Here's how the part is built. I have some questions about the finished solid (model axes, mm). A direction names the side the tool comes from. Give positions to 0.01 mm unless a question says otherwise; leave off trailing zeros. Write each loop counter-clockwise with the first axis right and the second up, starting at its lowest first coordinate (ties: lowest second). Pieces come first, ordered by that corner, then holes. Notation, with made-up numbers: (-26, 55) -> (-6, 55) arc R31 ccw to (-6, 80) -> close; hole circle Ø1 at (-26, -10.75). An arc over 180 degrees is marked (long way). Put each result on its own line as item: value. Start each with the question number.
Autodesk Inventor part; units mm, degrees
ref_plane "YZ Plane" through (0, 0, 0) normal (1, 0, 0) x (0, 1, 0)
ref_plane "XZ Plane" through (0, 0, 0) normal (0, 1, 0) x (-1, 0, 0)
ref_plane "XY Plane" through (0, 0, 0) normal (0, 0, 1) x (1, 0, 0)
sketch "Sketch1" plane through (0, 0, 0) normal (0, 0, 1) x (1, 0, 0)
  circle A0 centre (-24, 0) radius 1
  circle A1 centre (24, 0) radius 1
  circle A2 centre (-24, 0) radius 4
  circle A3 centre (24, 0) radius 4
  point P0 (0, 0)
  dimension "d0" = 2
  dimension "d1" = 2
  dimension "d3" = 48
  dimension "d4" = 24
  dimension "d5" = 8
  dimension "d6" = 8
extrude "Extrusion1" add sketch "Sketch1" against normal mid plane 18
sketch "Sketch2" plane through (0, 0, 0) normal (0, 0, 1) x (1, 0, 0)
  circle A0 centre (-24, 0) radius 4
  circle A1 centre (-24, 0) radius 1
  point P0 (0, 0)
extrude "Extrusion2" cut sketch "Sketch2" against normal mid plane 9
sketch "Sketch3" plane through (-24, 0, -4.5) normal (0, 0, 1) x (1, 0, 0)
  circle A0 centre (48, 0) radius 4
  circle A1 centre (48, 0) radius 4
  circle A2 centre (48, 0) radius 1
  point P0 (24, 0)
extrude "Extrusion3" cut sketch "Sketch3" against normal blind 4.5
mirror "Mirror1" about plane through (0, 0, 0) normal (0, 0, 1) of "Extrusion3"
sketch "Sketch6" plane through (0, 0, 0) normal (0, 1, 0) x (-1, 0, 0)
  line L0 (-20, -4.5) -> (-23, -4.5) construction
  line L1 (-23, -4.5) -> (-23, 4.5) construction
  line L2 (-23, 4.5) -> (-20, 4.5) construction
  line L3 (-20, 4.5) -> (-20, -4.5) construction
  line L4 (-25, -4.5) -> (-28, -4.5) construction
  line L5 (-28, -4.5) -> (-28, 4.5) construction
  line L6 (-28, 4.5) -> (-25, 4.5) construction
  line L7 (-25, 4.5) -> (-25, -4.5) construction
  line L8 (20, 9) -> (23, 9) construction
  line L9 (23, 9) -> (23, 4.5) construction
  line L10 (23, 4.5) -> (20, 4.5) construction
  line L11 (20, 4.5) -> (20, 9) construction
  line L12 (25, 9) -> (28, 9) construction
  line L13 (28, 9) -> (28, 4.5) construction
  line L14 (28, 4.5) -> (25, 4.5) construction
  line L15 (25, 4.5) -> (25, 9) construction
  line L16 (28, -9) -> (25, -9) construction
  line L17 (25, -9) -> (25, -4.5) construction
  line L18 (25, -4.5) -> (28, -4.5) construction
  line L19 (28, -4.5) -> (28, -9) construction
  line L20 (23, -9) -> (20, -9) construction
  line L21 (20, -9) -> (20, -4.5) construction
  line L22 (20, -4.5) -> (23, -4.5) construction
  line L23 (23, -4.5) -> (23, -9) construction
  line L24 (20, -9) -> (28, -9) construction
  line L25 (20, -9) -> (17, -9)
  line L26 (17, -9) -> (17, -2)
  line L27 (17, -2) -> (-20, -2)
  line L28 (-20, 4.5) -> (-20, -4.5) construction
  line L29 (-20, 2) -> (17, 2)
  line L30 (17, 2) -> (17, 9)
  line L31 (17, 9) -> (20, 9)
  line L32 (20, -4.5) -> (28, -4.5) construction
  line L33 (20, -4.5) -> (20, 4.5)
  line L34 (-20, -2) -> (-23, -2)
  line L35 (-23, -4.5) -> (-23, 4.5)
  line L36 (-20, 2) -> (-23, 2)
  line L37 (20, -9) -> (23, -9)
  line L38 (23, -4.5) -> (20, -4.5)
  line L39 (25, -4.5) -> (23, -4.5)
  line L40 (23, -4.5) -> (23, -9)
  line L41 (23, -9) -> (23, -4.5)
  line L42 (23, 4.5) -> (25, 4.5)
  line L43 (28, 4.5) -> (20, 4.5)
  line L44 (23, 4.5) -> (20, 4.5)
  line L45 (23, 9) -> (25, 9)
  line L46 (23, 4.5) -> (23, 9)
  line L47 (28, 9) -> (20, 9)
  line L48 (23, 9) -> (20, 9)
  point P0 (0, 0)
  dimension "d16" = 3
  dimension "d17" = 4
  dimension "d18" = 2
extrude "Extrusion4" add sketch "Sketch6" against normal mid plane 4
sketch "Sketch7" plane through (-20, -2, -4.5) normal (-1, 0, 0) x (0, 0, 1)
  circle A0 centre (4.5, 2) radius 1
  dimension "d21" = 2
extrude "Extrusion5" cut sketch "Sketch7" against normal blind 20
chamfer "Chamfer1" distance 1 angle 45 1 edges at (-20, 0, -1)
fillet "Fillet1" radius 2 4 edges at (1.7679, 2, 2) (1.7679, 2, -2) (1.7679, -2, -2) (1.7679, -2, 2)
sketch "Sketch9" plane through (0, 0, 9) normal (0, 0, 1) x (1, 0, 0)
  circle A0 centre (-24, 0) radius 1
  circle A1 centre (-24, 0) radius 0.9
  point P0 (0, 0)
  dimension "d29" = 1.8
extrude "TREAD" add sketch "Sketch9" against normal up to surface (4.5 mm away)
sketch "Sketch11" plane through (24, 0, 4.5) normal (0, 0, 1) x (1, 0, 0)
  circle A0 centre (0, 0) radius 4
  circle A1 centre (0, 0) radius 1
  point P0 (-24, 0)
extrude "thin" cut sketch "Sketch11" against normal blind 0.1
mirror "Mirror2" about plane through (0, 0, 0) normal (0, 0, 1) of "thin"
sketch "Sketch12" plane through (24, 0, 4.4) normal (0, 0, 1) x (1, 0, 0)
  circle A0 centre (0, 0) radius 1 construction
  circle A1 centre (0, 0) radius 1.1
  point P0 (-24, 0)
  dimension "d34" = 2.2
extrude "Extrusion8" cut sketch "Sketch12" against normal up to surface (8.8 mm away)
equation "\"d6\" = d5"
properties part number "Tolerenced_Phalalnge_48mm"
1) I want a section at B-B, the plane z = 7.25. Write out the boundary of the cut face in (x, y), and give its area (3 significant figures).
2) I want a section at D-D, the plane y = 2.75. Write out the boundary of the cut face in (x, z), and give its area (3 significant figures).
3) I want a section at C-C, the plane x = -24. Write out the boundary of the cut face in (y, z).
4) Which directions (+Z, -Z, +X, -X, +Y, -Y) give clear straight access to the entire face, cutting with the end or side of a thin tool? Please do faces 5 (the cylindrical face through (2.03, 1.4, -1.43)), 6 (the flat face through (-23, -1, -4.5)), 7 (the cylindrical face through (-10, -1, 0)), 8 (the flat face through (25, -1, 4.4)), 9 (the cylindrical face through (-25, 0, -7)).
5) I want a section at A-A, the plane x = 24. Write out the boundary of the cut face in (y, z), and give its area (3 significant figures).
6) Thinking about a two-plate mould opening in X: for faces 1 (the flat face through (-18, 2, 0)), 2 (the cylindrical face through (2.03, -1.43, -1.4)), 3 (the flat face through (-20, 0.5, -2.1)), 4 (the flat face through (-17, 0, 5)), which applies, released by +X, released by -X, zero draft, split by the parting line, or undercut?
7) I need wall thicknesses on probe 1 along Y at (x, z) = (-5.5, 0); probe 2 along Z at (x, y) = (-21.5, -1); probe 3 along Z at (x, y) = (1, 0). Which ranges of each line are inside material? Lowest first, please.
8) I'm going to push flat-ended pins straight in: pin 1 Ø4 at (x, y) = (22.5, 1.5) entering from +Z; pin 2 Ø5 at (x, z) = (9, 2) entering from +Y; pin 3 Ø10 at (x, z) = (-16.5, -4) entering from +Y; pin 4 Ø2 at (x, z) = (5.5, -4) entering from +Y. Where does each tip first touch, or does it pass through?
Established:
1. outline: (-20.54, -2) -> (-17, -2) -> (-17, 2) -> (-20.54, 2) arc R4 ccw (long way) to start; hole circle Ø1.8 at (-24, 0)
1. area: 60.4 mm2
2. outline: (-26.9, -9) -> (-21.1, -9) -> (-21.1, -4.5) -> (-26.9, -4.5) -> close; (-26.9, 4.5) -> (-21.1, 4.5) -> (-21.1, 9) -> (-26.9, 9) -> close; (21.1, -4.4) -> (26.9, -4.4) -> (26.9, 4.4) -> (21.1, 4.4) -> close
2. area: 103 mm2
3. outline: (-4, -9) -> (-1, -9) -> (-1, -4.5) -> (-4, -4.5) -> close; (-4, 4.5) -> (-0.9, 4.5) -> (-0.9, 9) -> (-4, 9) -> close; (0.9, 4.5) -> (4, 4.5) -> (4, 9) -> (0.9, 9) -> close; (1, -9) -> (4, -9) -> (4, -4.5) -> (1, -4.5) -> close
4. face 5: -Z, +Y
4. face 6: -X, +Y, -Y
4. face 7: -X
4. face 8: +Z, +X, +Y, -Y
4. face 9: -Z
5. outline: (-4, -4.4) -> (-1.1, -4.4) -> (-1.1, 4.4) -> (-4, 4.4) -> close; (1.1, -4.4) -> (4, -4.4) -> (4, 4.4) -> (1.1, 4.4) -> close
5. area: 51.0 mm2
6. face 1: zero draft
6. face 2: undercut
6. face 3: released by -X
6. face 4: undercut
7. probe 1: y = -2 to -1, 1 to 2
7. probe 2: z = -9 to -4.5, 4.5 to 9
7. probe 3: z = -2 to 2
8. pin 1: stops at z = 4.4
8. pin 2: stops at y = 2
8. pin 3: stops at y = 3.1
8. pin 4: passes through
